from build123d import *

# Parameters (mm, degrees)
SALIENTE_EXTRUIR1_DEPTH    = 28.75
REDONDEO1_R                = 5
REDONDEO2_R                = 10
REDONDEO3_R                = 1
CORTAR_EXTRUIR1_REACH      = 83.073
CROQUIS2_R                 = 3
CORTAR_EXTRUIR2_DEPTH      = 184.03816325
CORTAR_EXTRUIR2_DEPTH_BACK = 184.03816325
CROQUIS4_R                 = 5.999999992


with BuildPart() as part:
    # Croquis1 → Saliente-Extruir1 (new, symmetric)
    with BuildSketch(Plane.XY):
        Polygon((0, 33.5), (0, 0), (71.5, 0), (71.5, 3.5), (3.5, 3.5), (3.5, 33.5), align=None)
    extrude(amount=SALIENTE_EXTRUIR1_DEPTH, both=True)

    # Redondeo1
    redondeo1_edges = [part.edges().sort_by_distance(p)[0] for p in [
        (71.5, 1.75, -28.75),
        (71.5, 1.75, 28.75),
    ]]
    fillet(redondeo1_edges, radius=REDONDEO1_R)

    # Redondeo2
    redondeo2_edges = [part.edges().sort_by_distance(p)[0] for p in [
        (1.75, 33.5, 28.75),
        (1.75, 33.5, -28.75),
    ]]
    fillet(redondeo2_edges, radius=REDONDEO2_R)

    # Redondeo3
    redondeo3_edges = [part.edges().sort_by_distance(p)[0] for p in [
        (0, 0, 0),
        (3.5, 3.5, 0),
    ]]
    fillet(redondeo3_edges, radius=REDONDEO3_R)

    # Croquis2 → Cortar-Extruir1 (cut, up to next)
    with BuildSketch(Plane(origin=(3.5, 0, 0), x_dir=(0, 0, -1), z_dir=(1, 0, 0)), mode=Mode.PRIVATE) as cortar_extruir1_sk1:
        with Locations(Location((0, 17.5, 0), (0, 0, 90))):
            Circle(CROQUIS2_R)
    cortar_extruir1_tool1 = extrude(cortar_extruir1_sk1.sketch, amount=-CORTAR_EXTRUIR1_REACH, mode=Mode.PRIVATE) & part.part
    # Croquis2 → Cortar-Extruir1 (cut, up to next)
    with BuildSketch(Plane(origin=(3.5, 0, 0), x_dir=(0, 0, -1), z_dir=(1, 0, 0)), mode=Mode.PRIVATE) as cortar_extruir1_sk2:
        with Locations(Location((20, 17.5, 0), (0, 0, 90))):
            Circle(CROQUIS2_R)
    cortar_extruir1_tool2 = extrude(cortar_extruir1_sk2.sketch, amount=-CORTAR_EXTRUIR1_REACH, mode=Mode.PRIVATE) & part.part
    # Croquis2 → Cortar-Extruir1 (cut, up to next)
    with BuildSketch(Plane(origin=(3.5, 0, 0), x_dir=(0, 0, -1), z_dir=(1, 0, 0)), mode=Mode.PRIVATE) as cortar_extruir1_sk3:
        with Locations(Location((-20, 17.5, 0), (0, 0, 90))):
            Circle(CROQUIS2_R)
    cortar_extruir1_tool3 = extrude(cortar_extruir1_sk3.sketch, amount=-CORTAR_EXTRUIR1_REACH, mode=Mode.PRIVATE) & part.part
    add(cortar_extruir1_tool1.solids().sort_by_distance((3.5, 17.5, 0))[0], mode=Mode.SUBTRACT)
    add(cortar_extruir1_tool2.solids().sort_by_distance((3.5, 17.5, -20))[0], mode=Mode.SUBTRACT)
    add(cortar_extruir1_tool3.solids().sort_by_distance((3.5, 17.5, 20))[0], mode=Mode.SUBTRACT)

    # Croquis4 → Cortar-Extruir2 (cut, two sides: drawn at the far end of the back side and taken through both)
    with BuildSketch(Plane(origin=(-28.4, 19.037282969, -123.435876688), x_dir=(5.237222008265864e-15, 0.866025403784376, -0.5000000000001087), z_dir=(1, 0, 0)).offset(-CORTAR_EXTRUIR2_DEPTH_BACK)):
        with Locations(Location((-63.049264441, 106.129963469, 0), (0, 0, 120))):
            Circle(CROQUIS4_R)
    extrude(amount=CORTAR_EXTRUIR2_DEPTH + CORTAR_EXTRUIR2_DEPTH_BACK, mode=Mode.SUBTRACT)


solid = part.part
Model file for the job. Use its own axes, mm. A direction names the side the tool comes from. Coordinates: 2 decimals unless noted, no trailing zeros. Write each loop counter-clockwise with the first axis right and the second up, starting at its lowest first coordinate (ties: lowest second). Pieces come first, ordered by that corner, then holes. Notation, with made-up numbers: (8, -16.5) -> (62, -16.5) arc R22 cw to (62, -0.5) -> close; hole circle Ø7 at (48, 29). An arc over 180 degrees is marked (long way). One line per item, written item: value. Start each with the question number.
1) Slice it at D-D on x = 28. Write the cut outline in (y, z).
2) Probe probe 1 along Y at (x, z) = (1.8, 0); probe 2 along X at (y, z) = (32.5, 0); probe 3 along Z at (x, y) = (2, 17). List the from-to ranges inside material, lowest first.
3) Slice it at A-A on y = 17.5. Write the cut outline in (x, z), then the cut area to 3 significant figures.
4) Flat gauge pins, fed straight in: pin 1 Ø8 at (x, z) = (15, 2) entering from +Y; pin 2 Ø3.5 at (y, z) = (17.5, 20) entering from +X; pin 3 Ø12 at (y, z) = (27.5, 4.5) entering from -X. Where does each tip first touch, or does it go through?
5) Slice it at B-B on z = 0. Write the cut outline in (x, y).
6) Which spindle directions (+Z, -Z, +X, -X, +Y, -Y) get a long thin tool onto all of the face, cutting with end or side? Do faces 4 (the face through (38, 3.5, 0)), 5 (the face through (0, 17, 7)). Say none if no direction does.
7) Slice it at C-C on y = 13. Write the cut outline in (x, z), then the cut area to 3 significant figures.
8) Pull direction Y, two halves, no side cores. Call faces 1 (the face through (36, 0, 0)), 2 (the face through (3.5, 19, -6)), 3 (the face through (1.77, 16.85, -22.93)): +Y half, -Y half, draft (parallel to the pull), parting line (faces both ways), or undercut.
Answers follow:
1. outline: (0, -28.75) -> (3.5, -28.75) -> (3.5, 28.75) -> (0, 28.75) -> close
2. probe 1: 0 to 11.5, 23.5 to 33.5
2. probe 2: 0 to 3.5
2. probe 3: -28.75 to -22.96, -17.04 to -5.98, 5.98 to 17.04, 22.96 to 28.75
3. outline: (0, -28.75) -> (3.5, -28.75) -> (3.5, -23) -> (0, -23) -> close; (0, -17) -> (3.5, -17) -> (3.5, -6) -> (0, -6) -> close; (0, 6) -> (3.5, 6) -> (3.5, 17) -> (0, 17) -> close; (0, 23) -> (3.5, 23) -> (3.5, 28.75) -> (0, 28.75) -> close
3. area: 117 mm2
4. pin 1: y = 3.5
4. pin 2: through
4. pin 3: x = 0
5. outline: (0, 1) arc R1 ccw to (1, 0) -> (71.5, 0) -> (71.5, 3.5) -> (4.5, 3.5) arc R1 cw to (3.5, 4.5) -> (3.5, 11.5) -> (0, 11.5) -> close; (0, 23.5) -> (3.5, 23.5) -> (3.5, 33.5) -> (0, 33.5) -> close
6. face 4: +Z, -Z, +X, +Y
6. face 5: +Z, -Z, -X, +Y, -Y
7. outline: (0, -28.75) -> (3.5, -28.75) -> (3.5, -3.97) -> (0, -3.97) -> close; (0, 3.97) -> (3.5, 3.97) -> (3.5, 28.75) -> (0, 28.75) -> close
7. area: 173 mm2
8. face 1: -Y half
8. face 2: draft
8. face 3: undercut
